from build123d import *

# Parameters (mm, degrees)
SALIENTE_EXTRUIR1_DEPTH = 0.1


with BuildPart() as part:
    # Model → Saliente-Extruir1 (new body)
    with BuildSketch(Plane.XY):
        with BuildLine():
            Line((34.712434383, 29.082277171), (47.712434383, 29.082277171))
            ThreePointArc((47.712434383, 29.082277171), (48.419541165, 28.789383952), (48.712434383, 28.082277171))
            Line((48.712434383, 28.082277171), (48.712434383, -25.917722829))
            ThreePointArc((48.712434383, -25.917722829), (48.419541165, -26.62482961), (47.712434383, -26.917722829))
            Line((47.712434383, -26.917722829), (39.712434383, -26.917722829))
            ThreePointArc((39.712434383, -26.917722829), (39.005327602, -27.210616048), (38.712434383, -27.917722829))
            Line((38.712434383, -27.917722829), (38.712434383, -45.917722829))
            Line((38.712434383, -45.917722829), (20.548823016, -45.917722829))
            Line((20.548823016, -45.917722829), (20.548823016, -27.917722829))
            ThreePointArc((20.548823016, -27.917722829), (20.255929797, -27.210616048), (19.548823016, -26.917722829))
            Line((19.548823016, -26.917722829), (11.548823016, -26.917722829))
            ThreePointArc((11.548823016, -26.917722829), (10.841716234, -27.210616048), (10.548823016, -27.917722829))
            Line((10.548823016, -27.917722829), (10.548823016, -45.917722829))
            Line((10.548823016, -45.917722829), (-7.614788352, -45.917722829))
            Line((-7.614788352, -45.917722829), (-7.614788352, -28.139448744))
            ThreePointArc((-7.614788352, -28.139448744), (-7.907681571, -27.432341963), (-8.614788352, -27.139448744))
            Line((-8.614788352, -27.139448744), (-16.614788352, -27.139448744))
            ThreePointArc((-16.614788352, -27.139448744), (-17.321895133, -26.846555525), (-17.614788352, -26.139448744))
            Line((-17.614788352, -26.139448744), (-17.614788352, 28.082277171))
            ThreePointArc((-17.614788352, 28.082277171), (-17.321895133, 28.789383952), (-16.614788352, 29.082277171))
            Line((-16.614788352, 29.082277171), (-3.614788352, 29.082277171))
            Line((-3.614788352, 29.082277171), (34.712434383, 29.082277171))
        make_face()
        Polygon((31.548823016, 11.082277171), (31.548823016, -20.917722829), (-0.451176984, -20.917722829), (-0.451176984, 11.082277171), (16.048823016, 11.082277171), align=None, mode=Mode.SUBTRACT)
    extrude(amount=SALIENTE_EXTRUIR1_DEPTH)


solid = part.part
Can you work these out from the model? Positions are in its coordinate system, mm. Round coordinates to 2 decimals unless told otherwise and drop trailing zeros. Write each loop counter-clockwise with the first axis right and the second up, starting at its lowest first coordinate (ties: lowest second). Pieces come first, ordered by that corner, then holes. Notation, with made-up numbers: (-19.5, 72) -> (17.5, 72) arc R21 ccw to (17.5, 82) -> close; hole circle Ø2 at (-21.75, 26). An arc over 180 degrees is marked (long way). Use one line per item in the form item = value. Start each with the question number.
Q1. Imagine slicing it at A-A (x = 7). Please give me the cut outline in (y, z).
Q2. Imagine slicing it at B-B (y = -2.5). Please give me the cut outline in (x, z), then the cut area to 3 significant figures.
Q3. Imagine slicing it at D-D (x = -12). Please give me the cut outline in (y, z), then the cut area to 3 significant figures.
Q4. If I drill on probe 1 along Y at (x, z) = (42.5, 0.05), over which ranges is the centre line in solid material (lowest first)? Write a range as [from, to].
Q5. Imagine slicing it at C-C (z = 0.05). Please give me the cut outline in (x, y).
Q6. I'm going to push a flat-ended pin straight in: P1, Ø8, axis at x = 6, y = -14.5, coming from the +Z side. Where does the tip first touch, or does it pass through?
Worked out:
q1.outline = (-45.92, 0) -> (-20.92, 0) -> (-20.92, 0.1) -> (-45.92, 0.1) -> close; (11.08, 0) -> (29.08, 0) -> (29.08, 0.1) -> (11.08, 0.1) -> close
q2.outline = (-17.61, 0) -> (-0.45, 0) -> (-0.45, 0.1) -> (-17.61, 0.1) -> close; (31.55, 0) -> (48.71, 0) -> (48.71, 0.1) -> (31.55, 0.1) -> close
q2.area = 3.43 mm^2
q3.outline = (-27.14, 0) -> (29.08, 0) -> (29.08, 0.1) -> (-27.14, 0.1) -> close
q3.area = 5.62 mm^2
q4.probe_1 = [-26.92, 29.08]
q5.outline = (-17.61, -26.14) arc R1 ccw to (-16.61, -27.14) -> (-8.61, -27.14) arc R1 cw to (-7.61, -28.14) -> (-7.61, -45.92) -> (10.55, -45.92) -> (10.55, -27.92) arc R1 cw to (11.55, -26.92) -> (19.55, -26.92) arc R1 cw to (20.55, -27.92) -> (20.55, -45.92) -> (38.71, -45.92) -> (38.71, -27.92) arc R1 cw to (39.71, -26.92) -> (47.71, -26.92) arc R1 ccw to (48.71, -25.92) -> (48.71, 28.08) arc R1 ccw to (47.71, 29.08) -> (-16.61, 29.08) arc R1 ccw to (-17.61, 28.08) -> close; hole (-0.45, -20.92) -> (31.55, -20.92) -> (31.55, 11.08) -> (-0.45, 11.08) -> close
q6.P1 = through
